The figure shows three views and two pictorial views of one solid part (mm, origin at its lowest corner). Answer the questions. A direction names the side the tool comes from. Coordinates: 2 decimals unless noted, no trailing zeros. Order: outer loops, then holes, each group sorted by start corner. A loop starts at its lowest first (then second) coordinate and runs counter-clockwise, first axis right, second up. Notation, with made-up numbers: M -29.5,17.25 L 18.5,17.25 A28 ccw 18.5,52.25 Z; hole C 28,52.5 d6. An arc over 180 degrees is marked long. Write item = value, one per line. Start each with the question number.
Q1. Find section C-C on y = 1.5. Give the vertices of the cut face in (x, z), and give its area (3 significant figures).
Q2. Straight lines are drawn through the part: line 1 along Y through (x, z) = (18.5, 16); line 2 along X through (y, z) = (12.25, 12); line 3 along Z through (x, y) = (13.5, 11.5). For each, find the intervals that lie inside material, in ascending order.
Q3. Find section B-B on z = 34.5. Give the vertices of the cut face in (x, y), and give its area (3 significant figures).
Q4. Find section A-A on x = 10.25. Give the vertices of the cut face in (y, z).
Q5. Each of these flat-tipped pins is pushed along its axis until it touches: P1, Ø6.5, axis at y = 7.5, z = 14, coming from the -X side; P2, Ø4, axis at y = 7.5, z = 18.5, coming from the +X side; P3, Ø3, axis at x = 9, y = 5, coming from the -Z side. Where does it stop, or does it pass through?
Q6. Find section D-D on x = 2.5. Give the vertices of the cut face in (y, z), and give its area (3 significant figures).
Q7. A tool of negligible diameter and unlimited length cuts with its end or side. For the marked faces 1, 2, 3, 4 and 5, from which of +Z, -Z, +X, -X, +Y, -Y can it reach the whole face along a straight path? Write none if from no direction.
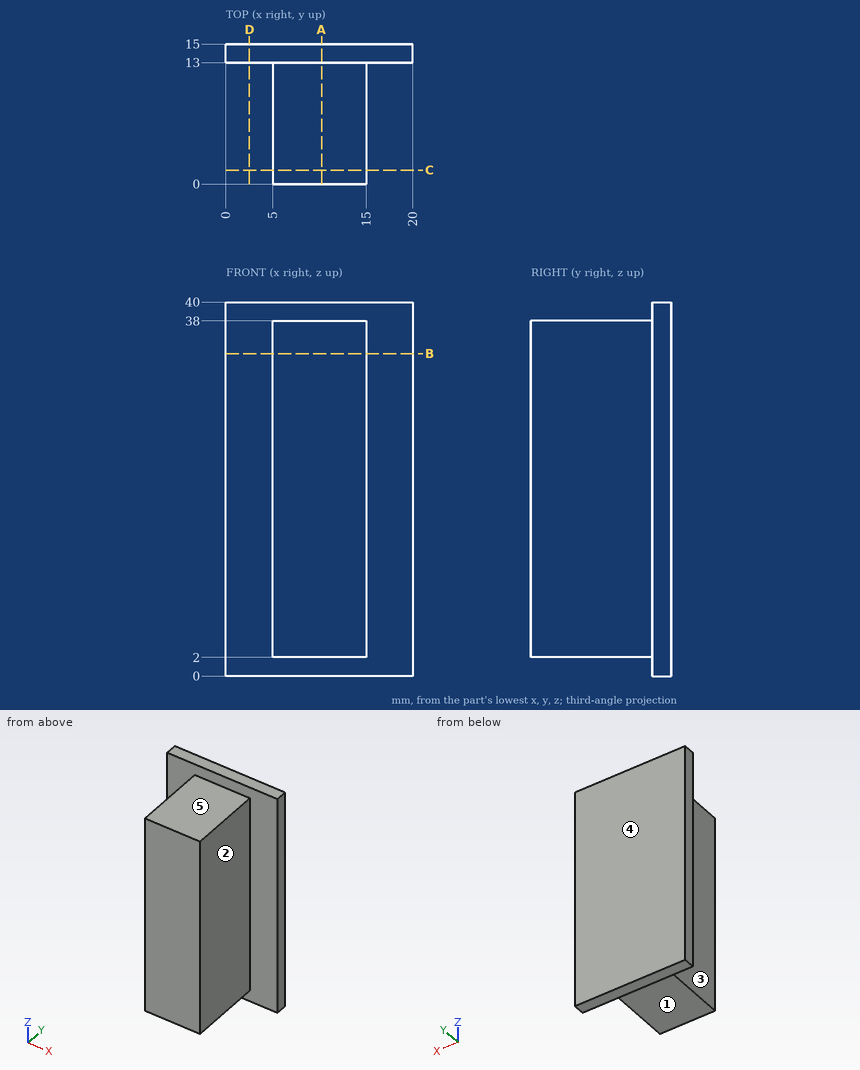
Findings below:
q1.outline = M 5,2 L 15,2 L 15,38 L 5,38 Z
q1.area = 360 mm^2
q2.line_1 = 13 to 15
q2.line_2 = 5 to 15
q2.line_3 = 2 to 38
q3.outline = M 0,13 L 5,13 L 5,0 L 15,0 L 15,13 L 20,13 L 20,15 L 0,15 Z
q3.area = 170 mm^2
q4.outline = M 0,2 L 13,2 L 13,0 L 15,0 L 15,40 L 13,40 L 13,38 L 0,38 Z
q5.P1 = 5
q5.P2 = 15
q5.P3 = 2
q6.outline = M 13,0 L 15,0 L 15,40 L 13,40 Z
q6.area = 80.0 mm^2
q7.face_1 = -Z, +X, -X, -Y
q7.face_2 = +Z, -Z, +X, -Y
q7.face_3 = +Z, -Z, -X, -Y
q7.face_4 = +Z, -Z, +X, -X, +Y
q7.face_5 = +Z, +X, -X, -Y
